Source: CAD feature listing. Evaluate the final solid. Frame: model axes, mm. A direction names the side the tool comes from. Round coordinates to 2 decimals unless told otherwise and drop trailing zeros. Write each loop counter-clockwise with the first axis right and the second up, starting at its lowest first coordinate (ties: lowest second). Pieces come first, ordered by that corner, then holes.
from build123d import *

# Parameters (mm, degrees)
SKETCH1_R                = 5
BOSS_EXTRUDE1_DEPTH      = 200
BOSS_EXTRUDE2_DEPTH      = 10
BOSS_EXTRUDE2_DEPTH_BACK = 10
SKETCH2_R                = 5
BOSS_EXTRUDE3_START      = 30
BOSS_EXTRUDE3_OUTLINE_R  = 6
BOSS_EXTRUDE3_DEPTH      = 10
BOSS_EXTRUDE4_START      = -10
SKETCH3_R                = 6
BOSS_EXTRUDE4_DEPTH      = 10


# Read off the part's stored shape, not the designer's step: Boss-Extrude3
with BuildPart() as part:
    # Sketch1 → Boss-Extrude1 (new body)
    with BuildSketch(Plane(origin=(0, 0, 0), x_dir=(1, 0, 0), z_dir=(0, 1, 0))):
        with Locations(Location((0, 0, 0), (0, 0, 270))):
            Circle(SKETCH1_R)
    extrude(amount=BOSS_EXTRUDE1_DEPTH)

    # Sketch2 → Boss-Extrude2 (add, two sides: drawn at the far end of the back side and taken through both)
    with BuildSketch(Plane.XY.offset(-BOSS_EXTRUDE2_DEPTH_BACK)):
        Circle(SKETCH2_R)
    extrude(amount=BOSS_EXTRUDE2_DEPTH + BOSS_EXTRUDE2_DEPTH_BACK)

    # Boss-Extrude3 outline → Boss-Extrude3 (add)
    with BuildSketch(Plane(origin=(0, 0, 0), x_dir=(1, 0, 0), z_dir=(0, 1, 0)).offset(BOSS_EXTRUDE3_START)):
        Circle(BOSS_EXTRUDE3_OUTLINE_R)
    extrude(amount=BOSS_EXTRUDE3_DEPTH)

    # Sketch3 → Boss-Extrude4 (add)
    with BuildSketch(Plane(origin=(0, 200, 0), x_dir=(1, 0, 0), z_dir=(0, 1, 0)).offset(BOSS_EXTRUDE4_START)):
        with Locations(Location((0, 0, 0), (0, 0, 270))):
            Circle(SKETCH3_R)
    extrude(amount=BOSS_EXTRUDE4_DEPTH)


solid = part.part
1) Section query B-B on x = 0. Return the cut outline in (y, z).
Taken from the geometry:
outline: (-5, -10) - (5, -10) - (5, -5) - (30, -5) - (30, -6) - (40, -6) - (40, -5) - (190, -5) - (190, -6) - (200, -6) - (200, 6) - (190, 6) - (190, 5) - (40, 5) - (40, 6) - (30, 6) - (30, 5) - (5, 5) - (5, 10) - (-5, 10) - close
2) Material intervals for line 1 (Y direction, x = 2.25, z = -4.5); line 2 (Z direction, x = 0.5, y = 143); line 3 (X direction, y = 181, z = 0.25), sorted ascending.
Taken from the geometry:
line 1: y = -4.47 to 4.47, 30 to 40, 190 to 200
line 2: z = -4.97 to 4.97
line 3: x = -4.99 to 4.99
3) Section query A-A on z = 0. Return the cut outline in (x, y), then the cut area to 3 significant figures.
Taken from the geometry:
outline: (-6, 30) - (-5, 30) - (-5, 0) arc R5 ccw to (5, 0) - (5, 30) - (6, 30) - (6, 40) - (5, 40) - (5, 190) - (6, 190) - (6, 200) - (-6, 200) - (-6, 190) - (-5, 190) - (-5, 40) - (-6, 40) - close
area: 2,080 mm2
4) Reachability of faces 1 (the face through (0, 0, 10)), 2 (the face through (4, 190, -4)), 3 (the face through (-6, 35, 0)) from +Z, -Z, +X, -X, +Y, -Y: full face, straight path, thin tool, end or side. Return the list, or none.
Taken from the geometry:
face 1: +Z, +X, -X, +Y, -Y
face 2: none
face 3: +Y
5) Pull-direction query (Y, two-part tool) for faces 4 (the face through (0, 200, 0)), 5 (the face through (0, 0, -10)), 6 (the face through (-4, 30, -4)); classes: released by +Y, released by -Y, zero draft, split by the parting line, or undercut.
Taken from the geometry:
face 4: released by +Y
face 5: zero draft
face 6: undercut
6) Section query C-C on y = 126. Return the cut outline in (x, z), then the cut area to 3 significant figures.
Taken from the geometry:
outline: circle Ø10 at (0, 0)
area: 78.5 mm2
7) Contact query for a flat-ended pin moving along its axis: P1, Ø2, axis at x = 0, y = 113, coming from the +Z side. Output: stop coordinate, or through.
Taken from the geometry:
P1: stops at z = 5
